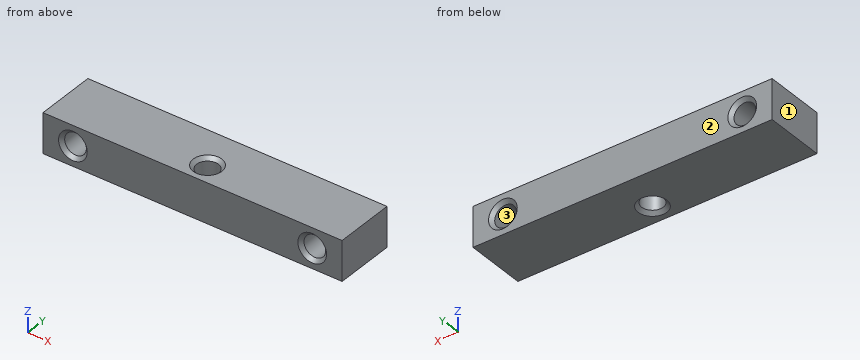
```python
from build123d import *

# Parameters (mm, degrees)
SKETCH1_W                      = 6.35
SKETCH1_H                      = 9.525
BOSS_EXTRUDE1_DEPTH            = 23.8125
F_8_32_TAPPED_HOLE1_AT_2_COUNT = 2
F_8_32_TAPPED_HOLE1_AT_2_PITCH = 38.1


with BuildPart() as part:
    # Sketch1 → Boss-Extrude1 (new, symmetric)
    with BuildSketch(Plane(origin=(0, 0, 0), x_dir=(0, 0, -1), z_dir=(1, 0, 0))):
        Rectangle(SKETCH1_W, SKETCH1_H)
    extrude(amount=BOSS_EXTRUDE1_DEPTH, both=True)

    # Sketch2 → #8-32 Tapped Hole1 (revolve, cut)
    with BuildSketch(Plane(origin=(19.05, 4.7625, 0), x_dir=(0, 0, 1), z_dir=(1, 0, 0))):
        Polygon((0, 0), (0, 9.525), (2.286, 9.525), (1.7272, 8.9662), (1.7272, 0.5588), (2.286, 0), align=None)
    f_8_32_tapped_hole1 = revolve(axis=Axis((19.05, 11.1125, 0), (0, -1, 0)), mode=Mode.SUBTRACT)

    # #8-32 Tapped Hole1 at 2: #8-32 Tapped Hole1 ×2
    with Locations(*[(-i * F_8_32_TAPPED_HOLE1_AT_2_PITCH, 0, 0) for i in range(1, F_8_32_TAPPED_HOLE1_AT_2_COUNT)]):
        add(f_8_32_tapped_hole1, mode=Mode.SUBTRACT)

    # Sketch4 → #8-32 Tapped Hole2 (revolve, cut)
    with BuildSketch(Plane(origin=(0, -1.5875, 3.175), x_dir=(0, -1, 0), z_dir=(1, 0, 0))):
        Polygon((0, 0), (0, 6.35), (2.286, 6.35), (1.7272, 5.7912), (1.7272, 0.5588), (2.286, 0), align=None)
    revolve(axis=Axis((0, -1.5875, 9.525), (0, 0, -1)), mode=Mode.SUBTRACT)


solid = part.part
```
Input: part model. Units: mm. Frame: model coordinates. Face numbers are marked on the shaded views. Give positions to 0.01 mm unless a question says otherwise; leave off trailing zeros. Order: outer loops, then holes, each group sorted by start corner. A loop starts at its lowest first (then second) coordinate and runs counter-clockwise, first axis right, second up.
1. Section D-D on x = 0. Return the cut outline in (y, z) (1 decimal).
Derived:
outline: (-4.8, -3.2) - (-3.9, -3.2) - (-3.3, -2.6) - (-3.3, 2.6) - (-3.9, 3.2) - (-4.8, 3.2) - close; (0.1, -2.6) - (0.7, -3.2) - (4.8, -3.2) - (4.8, 3.2) - (0.7, 3.2) - (0.1, 2.6) - close
2. Pin query (flat end, axial travel): pin 1 (4 mm diameter, centred on x = 0, y = -1.59, fed in from -Z). Return the tip coordinate at first contact, or that it passes through.
Derived:
pin 1: stops at z = -2.89
3. Section B-B on x = 19.05. Return the cut outline in (y, z) (1 decimal).
Derived:
outline: (-4.8, -3.2) - (4.8, -3.2) - (4.8, -2.3) - (4.2, -1.7) - (-4.2, -1.7) - (-4.8, -2.3) - close; (-4.8, 2.3) - (-4.2, 1.7) - (4.2, 1.7) - (4.8, 2.3) - (4.8, 3.2) - (-4.8, 3.2) - close
4. Section C-C on y = -1.75. Give the number of separate pieces and of enclosed holes in the cut face, and give its area (3 significant figures).
Derived:
separate pieces: 2
enclosed holes: 2
area: 261 mm2
5. Section A-A on z = 0. Return the cut outline in (x, y).
Derived:
outline: (-23.81, -4.76) - (-21.34, -4.76) - (-20.78, -4.2) - (-20.78, 4.2) - (-21.34, 4.76) - (-23.81, 4.76) - close; (-17.32, -4.2) - (-16.76, -4.76) - (16.76, -4.76) - (17.32, -4.2) - (17.32, 4.2) - (16.76, 4.76) - (-16.76, 4.76) - (-17.32, 4.2) - close; (20.78, -4.2) - (21.34, -4.76) - (23.81, -4.76) - (23.81, 4.76) - (21.34, 4.76) - (20.78, 4.2) - close; hole circle Ø3.45 at (0, -1.59)
6. Material intervals for L1, parallel to X at y = 1, z = 0; L2, parallel to X at y = -1.5, z = 0; L3, parallel to Y at x = 0, z = 0.9, sorted ascending.
Derived:
L1: x = -23.81 to -20.78, -17.32 to 17.32, 20.78 to 23.81
L2: x = -23.81 to -20.78, -17.32 to -1.72, 1.72 to 17.32, 20.78 to 23.81
L3: y = -4.76 to -3.31, 0.14 to 4.76
7. Mould query, pull axis X, two halves, no side actions, for the marked faces 1, 2 and 3. Classes: released by +X, released by -X, zero draft, split by the parting line, or undercut.
Derived:
face 1: released by -X
face 2: zero draft
face 3: undercut
